Study the drawing (mm; zero at the part's minimum x, y, z) and answer. Coordinates: 2 decimals unless noted, no trailing zeros. Order: outer loops, then holes, each group sorted by start corner. A loop starts at its lowest first (then second) coordinate and runs counter-clockwise, first axis right, second up. Notation, with made-up numbers: (-33.75, -8.75) -> (-0.75, -8.75) arc R16 cw to (-0.75, 1.25) -> close; hole circle Ø6 at (6, 59.25). An arc over 180 degrees is marked (long way). One line per question, with ' | ' between items.
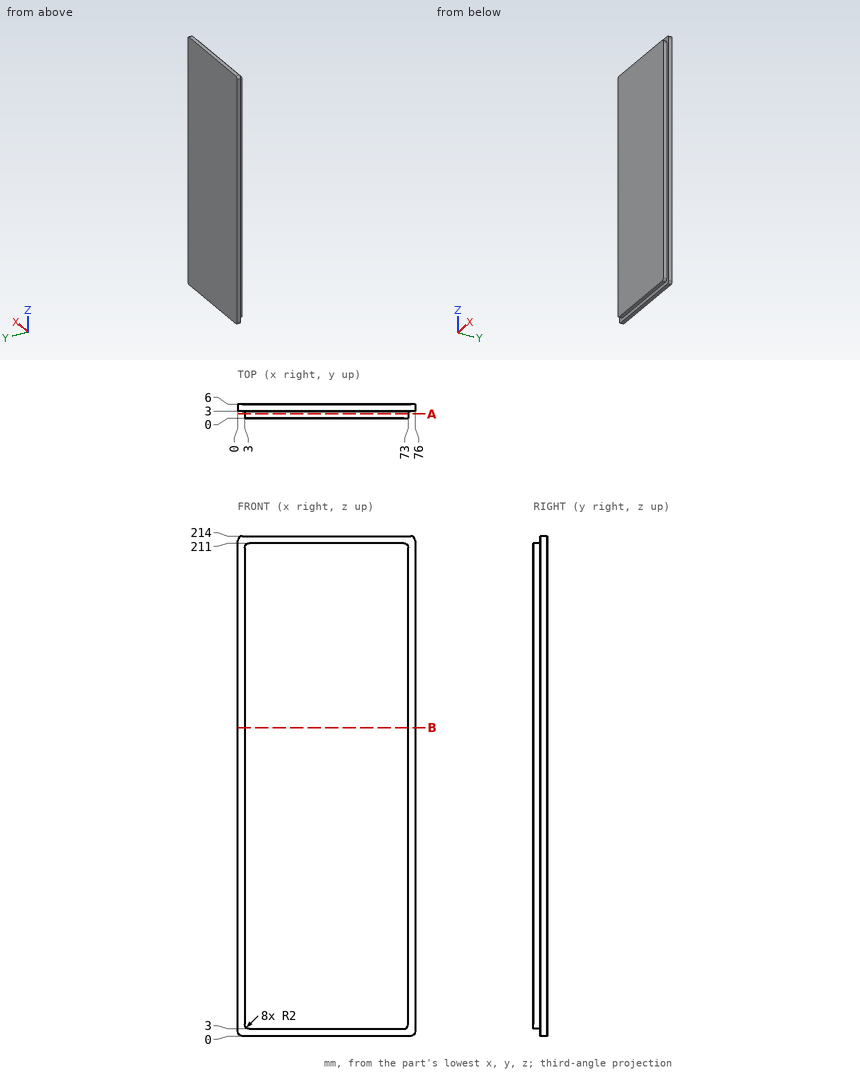
Item 1: Section A-A, the plane y = 1.75 is taken. Give the vertices of the cut face in (x, z).
Computed values:
outline: (3, 5) arc R2 ccw to (5, 3) -> (71, 3) arc R2 ccw to (73, 5) -> (73, 209) arc R2 ccw to (71, 211) -> (5, 211) arc R2 ccw to (3, 209) -> close
Item 2: Each of these flat-tipped pins is pushed along its axis until it touches: pin 1 Ø0.9 at (y, z) = (1, 112) entering from +X; pin 2 Ø2 at (y, z) = (1.5, 184) entering from -X; pin 3 Ø0.9 at (x, y) = (49.5, 2) entering from +Z. Where does it stop, or does it pass through?
Computed values:
pin 1: stops at x = 73 | pin 2: stops at x = 3 | pin 3: stops at z = 211
Item 3: Find the intervals of material crossed by L1, parallel to Z at x = 28.5, y = 0.95; L2, parallel to X at y = 0.8, z = 102; L3, parallel to Z at x = 3.5, y = 0.7, in increasing order.
Computed values:
L1: z = 3 to 211 | L2: x = 3 to 73 | L3: z = 3.68 to 210.32
Item 4: Section B-B, the plane z = 132 is taken. Give the vertices of the cut face in (x, y).
Computed values:
outline: (0, 3) -> (3, 3) -> (3, 0) -> (73, 0) -> (73, 3) -> (76, 3) -> (76, 6) -> (0, 6) -> close
